from build123d import *

# Parameters (mm, degrees)
EXTRUDE_1_OUTLINE_R   = 2
EXTRUDE_1_OUTLINE_R_2 = 22.5
EXTRUDE_1_OUTLINE_R_3 = 11.5
EXTRUDE_1_DEPTH       = 3
EXTRUDE_START         = 1
SKETCH_2_3_R          = 11.5
SKETCH_2_3_R_2        = 8.5
EXTRUDE_2_DEPTH       = 2
HOLE_WIZARD_M3_1_D    = 2.5


# Read off the part's stored shape, not the designer's step: the extrude step
with BuildPart() as part:
    # Extrude 1 outline → Extrude 1 (new body)
    with BuildSketch(Plane.XY):
        with BuildLine():
            Line((-248.314941285, 75.355462585), (-108.600675895, 22.676132978))
            ThreePointArc((-108.600675895, 22.676132978), (-55.335467517, 50.642415933), (-89.342878346, 100.2689352))
            Line((-89.342878346, 100.2689352), (-237.47523438, 119.030406823))
            ThreePointArc((-237.47523438, 119.030406823), (-264.732559951, 102.612788156), (-248.314941285, 75.355462585))
        make_face()
        with Locations((-122.546352319, 67.32352005)):
            Circle(EXTRUDE_1_OUTLINE_R, mode=Mode.SUBTRACT)
        with Locations((-94.40027703, 60.337932808)):
            Circle(EXTRUDE_1_OUTLINE_R_2, mode=Mode.SUBTRACT)
        with Locations((-242.895087832, 97.192934704)):
            Circle(EXTRUDE_1_OUTLINE_R_3, mode=Mode.SUBTRACT)
    extrude(amount=EXTRUDE_1_DEPTH)

    # Sketch 2_3 → Extrude 2 (add)
    with BuildSketch(Plane.XY.offset(EXTRUDE_START)):
        with Locations((-242.895087832, 97.192934704)):
            Circle(SKETCH_2_3_R)
        with Locations((-242.895087832, 97.192934704)):
            Circle(SKETCH_2_3_R_2, mode=Mode.SUBTRACT)
    extrude(amount=EXTRUDE_2_DEPTH)

    # Hole Wizard M3 _1 (through all)
    with Locations(Plane.XY.offset(3)):
        with Locations((-79.183536118, 94.611841193), (-60.712733566, 76.812137352), (-58.004707111, 51.303968462), (-72.326572251, 30.022892769), (-96.97696912, 22.926562105), (-120.421703236, 33.33542592), (-131.690722835, 56.379062808), (-125.511128404, 81.275098967), (-104.774420857, 96.374402389)):
            Hole(HOLE_WIZARD_M3_1_D / 2)


solid = part.part
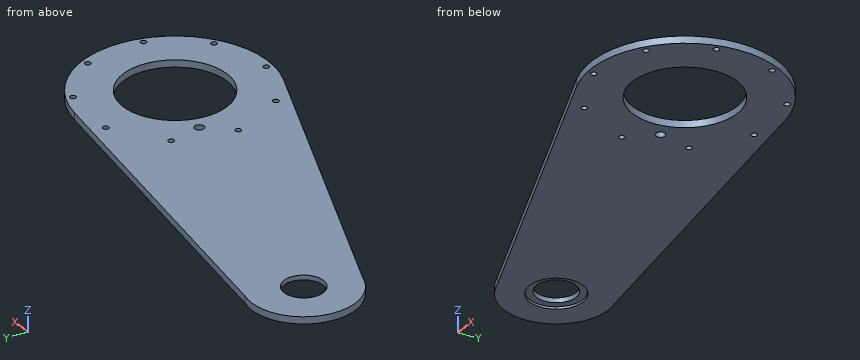
Input: part model. Units: mm. Frame: model coordinates. Give positions to 0.01 mm unless a question says otherwise; leave off trailing zeros. Loops run counter-clockwise (first coordinate to the right, second up) from the corner with the lowest first, then second, coordinate; pieces in that order, holes last. Notation, with made-up numbers: (66, -37.5) -> (120, -37.5) arc R26 cw to (120, -9.5) -> close; hole circle Ø4 at (81, 12). An arc over 180 degrees is marked (long way). Answer as a JSON object with one key per item and string values. Group by question number.
Item 1: Cut plane D-D, the plane y = 41.5. Return the cut outline in (x, z).
Item 2: Cut plane C-C, the plane x = -243. Return the cut outline in (y, z).
Item 3: Cut plane A-A, the plane y = 63. Return the cut outline in (x, z), and give its area (3 significant figures).
Item 4: Cut plane B-B, the plane z = 1.75. State how many separate pieces and enclosed holes the cut face has, and give its area (3 significant figures).
Item 5: Pin query (flat end, axial travel): P1, Ø1.5, axis at x = -187, z = 1.5, coming from the +Y side. Return the tip coordinate at first contact, or that it passes through.
Item 6: Line query: probe 1 along X at (y, z) = (96, 0.1); probe 2 along Y at (x, z) = (-142, 1.6); probe 3 along Y at (x, z) = (-239, 2). Output: solid intervals per line, ascending.
Checks:
{
 "1": {"outline": "(-158.52, 0) -> (-106.7, 0) -> (-106.7, 3) -> (-158.52, 3) -> close; (-82.1, 0) -> (-58.83, 0) -> (-58.83, 3) -> (-82.1, 3) -> close"},
 "2": {"outline": "(73.35, 0) -> (85.69, 0) -> (85.69, 1) -> (88.69, 1) -> (88.69, 3) -> (73.35, 3) -> close; (105.69, 1) -> (108.69, 1) -> (108.69, 0) -> (119.69, 0) -> (119.69, 3) -> (105.69, 3) -> close"},
 "3": {"outline": "(-215.55, 0) -> (-116.74, 0) -> (-116.74, 3) -> (-215.55, 3) -> close; (-72.06, 0) -> (-54.24, 0) -> (-54.24, 3) -> (-72.06, 3) -> close", "area": "350 mm²"},
 "4": {"separate pieces": "1", "enclosed holes": "12", "area": "11,100 mm²"},
 "5": {"P1": "stops at y = 112.73"},
 "6": {"probe 1": "x = -265.36 to -254.33, -231.46 to -105.97, -103.58 to -75.74", "probe 2": "y = 35.27 to 106.94", "probe 3": "y = 71.84 to 89.64, 104.75 to 119.35"}
}
